```python
from build123d import *

# Parameters (mm, degrees)
SKETCH1_W               = 111.76
SKETCH1_H               = 3.302
SKETCH6_W               = 2.54
SKETCH6_H               = 4.318
CUT_EXTRUDE1_DEPTH      = 57.909605516
CUT_EXTRUDE1_DEPTH_BACK = 57.909605516
SKETCH7_W               = 7.62
SKETCH7_H               = 15.24
SKETCH8_W               = 55.88
SKETCH8_H               = 15.24
CUT_EXTRUDE2_DEPTH      = 57.909605516


with BuildPart() as part:
    # Sketch1 → Revolve1 (revolve)
    with BuildSketch(Plane.XY, mode=Mode.PRIVATE) as revolve1_sk:
        with Locations((0, 1.651)):
            Rectangle(SKETCH1_W, SKETCH1_H)
    revolve(revolve1_sk.sketch.rotate(Axis((-55.88, 0, 0), (1, 0, 0)), 90), axis=Axis((-55.88, 0, 0), (1, 0, 0)))

    # Sketch6 → Revolve2 (revolve)
    with BuildSketch(Plane.XY, mode=Mode.PRIVATE) as revolve2_sk:
        with Locations((-26.67, 5.461)):
            Rectangle(SKETCH6_W, SKETCH6_H)
        with Locations((26.67, 5.461)):
            Rectangle(SKETCH6_W, SKETCH6_H)
        with Locations((-54.61, 5.461)):
            Rectangle(SKETCH6_W, SKETCH6_H)
        with Locations((54.61, 5.461)):
            Rectangle(SKETCH6_W, SKETCH6_H)
    revolve(revolve2_sk.sketch.rotate(Axis((-31.878421892, 0, 0), (1, 0, 0)), 90), axis=Axis((-31.878421892, 0, 0), (1, 0, 0)))

    # Sketch7 → Cut-Extrude1 (cut, two sides: drawn at the far end of the back side and taken through both)
    with BuildSketch(Plane(origin=(0, 0, 0), x_dir=(0, 0, -1), z_dir=(1, 0, 0)).offset(-CUT_EXTRUDE1_DEPTH_BACK)):
        with Locations((3.81, 0)):
            Rectangle(SKETCH7_W, SKETCH7_H)
    extrude(amount=CUT_EXTRUDE1_DEPTH + CUT_EXTRUDE1_DEPTH_BACK, mode=Mode.SUBTRACT)

    # Sketch8 → Cut-Extrude2 (cut, through all)
    with BuildSketch(Plane.XY):
        with Locations((-27.94, 0)):
            Rectangle(SKETCH8_W, SKETCH8_H)
    extrude(amount=CUT_EXTRUDE2_DEPTH, mode=Mode.SUBTRACT)


solid = part.part
```
Here's how the part is built. I have some questions about the finished solid (model axes, mm). A direction names the side the tool comes from. Round coordinates to 2 decimals unless told otherwise and drop trailing zeros. Order: outer loops, then holes, each group sorted by start corner. A loop starts at its lowest first (then second) coordinate and runs counter-clockwise, first axis right, second up. Notation, with made-up numbers: M 37,-39.75 L 85,-39.75 A30 ccw 85,-3.75 Z; hole C 5.5,14 d1. An arc over 180 degrees is marked long. Answer in a Markdown table with one row per item.
Item 1: Imagine slicing it at D-D, the plane x = 51. Write out the boundary of the cut face in (y, z).
A:
| item | result |
|---|---|
| outline | M -3.3,0 L 3.3,0 A3.3 ccw Z |
Item 2: Imagine slicing it at C-C, the plane y = 0. Write out the boundary of the cut face in (x, z).
A:
| item | result |
|---|---|
| outline | M 0,0 L 55.88,0 L 55.88,7.62 L 53.34,7.62 L 53.34,3.3 L 27.94,3.3 L 27.94,7.62 L 25.4,7.62 L 25.4,3.3 L 0,3.3 Z |
Item 3: Imagine slicing it at B-B, the plane y = -4.5. Write out the boundary of the cut face in (x, z).
A:
| item | result |
|---|---|
| outline | M 25.4,0 L 27.94,0 L 27.94,6.15 L 25.4,6.15 Z; M 53.34,0 L 55.88,0 L 55.88,6.15 L 53.34,6.15 Z |
Item 4: If I drill on L1, parallel to X at y = 2.25, z = 3.5; L2, parallel to Z at x = 41, y = 0; L3, parallel to Z at x = 8.5, y = 3, over which ranges is the centre line in solid material (lowest first)? Write a range as from..to.
A:
| item | result |
|---|---|
| L1 | x = 25.4..27.94, 53.34..55.88 |
| L2 | z = 0..3.3 |
| L3 | z = 0..1.38 |
Item 5: For faces 1 (the face through (25.4, 0, 4)), 2 (the face through (28, 0, 0)), 3 (the face through (27.94, 0, 4)), which set-ups out of +Z, -Z, +X, -X, +Y, -Y let a thin tool reach every point of the face, with its end or its side?
A:
| item | result |
|---|---|
| face 1 | +Z, -X |
| face 2 | -Z, +X, -X, +Y, -Y |
| face 3 | +Z |
Item 6: I'm going to push flat-ended pins straight in: pin 1 (2.5 mm diameter, centred on y = 2.5, z = 4.5, fed in from -X); pin 2 (4 mm diameter, centred on x = 17, z = 3.5, fed in from +Y); pin 3 (3 mm diameter, centred on x = 22.5, z = 3.5, fed in from -Y). Where does each tip first touch, or does it pass through?
A:
| item | result |
|---|---|
| pin 1 | stops at x = 25.4 |
| pin 2 | stops at y = 2.94 |
| pin 3 | stops at y = -2.63 |
Item 7: Thinking about a two-plate mould opening in X: for faces 4 (the face through (54.63, 0.17, 7.62)), 5 (the face through (40.8, 0.1, 3.3)), 6 (the face through (55.88, 0, 3)), 7 (the face through (53.34, 0, 4)), which applies, +X half, -X half, draft (parallel to the pull), parting line (faces both ways), or undercut?
A:
| item | result |
|---|---|
| face 4 | draft |
| face 5 | undercut |
| face 6 | +X half |
| face 7 | undercut |
Item 8: Imagine slicing it at A-A, the plane z = 4. Write out the boundary of the cut face in (x, y), and give its area (3 significant figures).
A:
| item | result |
|---|---|
| outline | M 25.4,-6.49 L 27.94,-6.49 L 27.94,6.49 L 25.4,6.49 Z; M 53.34,-6.49 L 55.88,-6.49 L 55.88,6.49 L 53.34,6.49 Z |
| area | 65.9 mm2 |
